For this review, take the finished solid that the model builds, in its own axes (mm). Give positions to 0.01 mm unless a question says otherwise; leave off trailing zeros. Loops run counter-clockwise (first coordinate to the right, second up) from the corner with the lowest first, then second, coordinate; pieces in that order, holes last. Notation, with made-up numbers: (-33, 70) - (22, 70) arc R16 cw to (22, 78) - close; hole circle Ø4 at (-19.75, 38.25). An arc over 180 degrees is marked (long way). Answer in a Markdown table with one row per item.
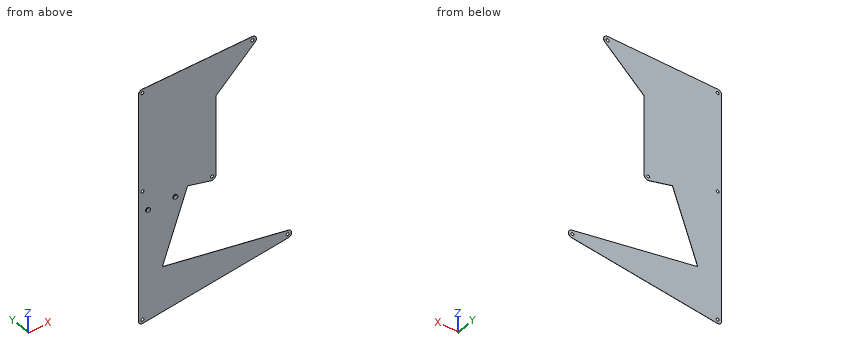
Autodesk Inventor part; units mm, degrees
ref_plane "Work Plane1" through (-205, 0.2, 0) normal (0, 1, 0) x (1, 0, 0)
ref_plane "Work Plane2" through (-205, 0.4, 0) normal (0, 1, 0) x (1, 0, 0)
ref_plane "YZ Plane" through (0, 0, 0) normal (1, 0, 0) x (0, 1, 0)
ref_plane "Work Plane1" through (-205, 0.2, 0) normal (0, 1, 0) x (1, 0, 0)
sketch "Sketch1" plane through (-205, 0.2, 0) normal (0, 1, 0) x (1, 0, 0)
  circle A0 centre (172.5, -37.3) radius 1.675
  circle A1 centre (172.5, -37.3) radius 4.5
  circle A2 centre (172.5, -37.3) radius 1.675
  circle A3 centre (7.5, -19) radius 1.675
  circle A4 centre (7.5, -19) radius 4.5
  circle A5 centre (7.5, -19) radius 1.675
  circle A6 centre (86.5, -146.2) radius 1.675
  circle A7 centre (86.5, -146.2) radius 4.5
  circle A8 centre (86.5, -146.2) radius 1.675
  circle A9 centre (7.5, -167.45) radius 1.675
  circle A10 centre (7.5, -167.45) radius 4.5
  circle A11 centre (7.5, -167.45) radius 1.675
  circle A12 centre (7.5, -281.46) radius 1.675
  circle A13 centre (7.5, -281.46) radius 4.5
  circle A14 centre (7.5, -281.46) radius 1.675
  circle A15 centre (132.5, -281.46) radius 1.675
  circle A16 centre (132.5, -281.46) radius 4.5
  circle A17 centre (132.5, -281.46) radius 1.675
  line L0 (132.5, -285.96) -> (7.5, -285.96)
  line L1 (3, -281.46) -> (3, -167.45)
  line L2 (135.7704, -278.369) -> (10.5327, -164.1254)
  line L3 (91, -146.2) -> (91, -237.5288)
  line L4 (84.825, -142.0234) -> (6.3328, -163.104)
  line L5 (91, -237.5288) -> (10.5327, -164.1254)
  line L6 (12, -19) -> (58.7973, -149.0136)
  line L7 (3, -19) -> (3, -167.45)
  line L8 (172.5, -41.8) -> (30.084, -69.2416)
  line L9 (172.5, -32.8) -> (8.061, -14.5351)
  point P0 (205, 0)
  dimension "d1" = 9
  dimension "d2" = 9
  dimension "d3" = 9
  dimension "d4" = 9
  dimension "d5" = 9
  dimension "d6" = 9
extrude "Extrusion1" add sketch "Sketch1" along normal blind 0.2 contours A1 | A1 L8 L6 A4 L9 | A4 | L6 L4 A10 L7 A4 | L4 A7 L3 L2 A10 | A10 | A10 L2 A16 L0 A13 L1 | A7 | A13 | A16 L2 picked at (134.365, -278.4554)
ref_plane "Work Plane2" through (-205, 0.4, 0) normal (0, 1, 0) x (1, 0, 0)
sketch "Sketch3" plane through (-205, 0.2, 0) normal (0, -1, 0) x (1, 0, 0)
  line L0 (3, 19) -> (3, 281.46)
  line L1 (3, 143.5142) -> (56.8178, 143.5142)
  line L2 (58.7973, 149.0136) -> (30.084, 69.2416)
  circle A0 centre (13.4848, 143.5142) radius 2.5
  circle A1 centre (44.4406, 143.5142) radius 2.5
  point P0 (205, 0)
  dimension "d11" = 5
  dimension "d12" = 5
extrude "Extrusion2" add sketch "Sketch3" along normal blind 1
properties part number "base_main_pcb_full"
1. We need section B-B, the plane y = -0.5. Give the boundary of the cut face in (x, z).
Values:
| item | result |
|---|---|
| outline | circle Ø5 at (-191.52, 143.51); circle Ø5 at (-160.56, 143.51) |
2. We need section C-C, the plane x = -95. Give the boundary of the cut face in (y, z).
Values:
| item | result |
|---|---|
| outline | (0.2, 25.86) - (0.4, 25.86) - (0.4, 53.84) - (0.2, 53.84) - close; (0.2, 254.86) - (0.4, 254.86) - (0.4, 285.96) - (0.2, 285.96) - close |
3. We need section A-A, the plane x = -134.5. Give the boundary of the cut face in (y, z), and give its area (3 significant figures).
Values:
| item | result |
|---|---|
| outline | (0.2, 21.47) - (0.4, 21.47) - (0.4, 61.45) - (0.2, 61.45) - close; (0.2, 145.87) - (0.4, 145.87) - (0.4, 285.96) - (0.2, 285.96) - close |
| area | 36.0 mm^2 |
4. Wall thickness on line 1 (X direction, y = 0.3, z = 281.46) (3 decimals); line 2 (Z direction, x = -197.5, y = 0.35) (3 decimals); line 3 (X direction, y = 0.3, z = 167.45) (3 decimals): over which ranges is each line inside the solid? List them lowest first. Write a range as [from, to].
Values:
| item | result |
|---|---|
| line 1 | x = [-202, -199.175], [-195.825, -74.175], [-70.825, -68] |
| line 2 | z = [14.5, 17.325], [20.675, 165.775], [169.125, 279.785], [283.135, 285.96] |
| line 3 | x = [-202, -199.175], [-195.825, -114] |
5. Clearance check with flat-ended pins moving along their axes: pin 1 (4.5 mm diameter, centred on x = -197.5, z = 167.45, fed in from -Y); pin 2 (2 mm diameter, centred on x = -118.5, z = 146.2, fed in from -Y). State where each tip first meets the part, or that it passes through.
Values:
| item | result |
|---|---|
| pin 1 | stops at y = 0.2 |
| pin 2 | passes through |
6. We need section D-D, the plane z = 131. Give the boundary of the cut face in (x, y).
Values:
| item | result |
|---|---|
| outline | (-202, 0.2) - (-152.69, 0.2) - (-152.69, 0.4) - (-202, 0.4) - close |
